```python
from build123d import *

# Parameters (mm, degrees)
SKETCH1_R               = 6.35
BOSS_EXTRUDE1_DEPTH     = 5.4
HORN_DEPTH              = 2.5
SKETCH4_R               = 1.4
CUT_EXTRUDE1_DEPTH      = 6.4
SKETCH5_R               = 0.5
CUT_EXTRUDE2_DEPTH      = 6.4
LPATTERN1_COUNT         = 4
LPATTERN1_PITCH         = 3
MIRROR1_COPY_1_SKETCH_R = 0.5
MIRROR1_COPY_1_DEPTH    = 6.4
MIRROR1_COPY_2_SKETCH_R = 0.5
MIRROR1_COPY_2_DEPTH    = 6.4
MIRROR1_COPY_3_SKETCH_R = 0.5
MIRROR1_COPY_3_DEPTH    = 6.4
CUT_EXTRUDE4_DEPTH      = 3
CIRPATTERN2_COUNT       = 26
SKETCH9_R               = 2.6
CUT_EXTRUDE5_DEPTH      = 3
SKETCH10_R              = 6.35
SKETCH10_R_2            = 4.25
CUT_EXTRUDE6_DEPTH      = 2.9
BOSS_EXTRUDE5_DEPTH     = 0.5
CIRPATTERN3_COUNT       = 4
SKETCH12_R              = 4.375
CUT_EXTRUDE7_DEPTH      = 1
SKETCH13_R              = 3.375
SKETCH13_R_2            = 2.875
BOSS_EXTRUDE6_DEPTH     = 1
SKETCH14_R              = 3.375
SKETCH14_R_2            = 2.875
BOSS_EXTRUDE7_DEPTH     = 0.35


with BuildPart() as part:
    # Sketch1 → Boss-Extrude1 (new body)
    with BuildSketch(Plane(origin=(0, 0, 0), x_dir=(1, 0, 0), z_dir=(0, 1, 0))):
        Circle(SKETCH1_R)
    extrude(amount=BOSS_EXTRUDE1_DEPTH)

    # Sketch2 → horn (add)
    with BuildSketch(Plane(origin=(0, 5.4, 0), x_dir=(1, 0, 0), z_dir=(0, 1, 0))):
        with BuildLine():
            Line((-2.609740545, 16.990167671), (-4.891612682, 4.049027706))
            ThreePointArc((-4.891612682, 4.049027706), (0, 6.35), (4.891612682, 4.049027706))
            Line((4.891612682, 4.049027706), (2.609740545, 16.990167671))
            ThreePointArc((2.609740545, 16.990167671), (0, 19.18), (-2.609740545, 16.990167671))
        make_face()
    horn = extrude(amount=-HORN_DEPTH)

    # Sketch4 → Cut-Extrude1 (cut, through all)
    with BuildSketch(Plane(origin=(0, 5.4, 0), x_dir=(-1, 0, 0), z_dir=(0, -1, 0))):
        Circle(SKETCH4_R)
    extrude(amount=CUT_EXTRUDE1_DEPTH, mode=Mode.SUBTRACT)

    # Sketch5 → Cut-Extrude2 (cut, through all)
    with BuildSketch(Plane(origin=(0, 0, 0), x_dir=(-1, 0, 0), z_dir=(0, -1, 0))):
        with Locations((0, 16.53)):
            Circle(SKETCH5_R)
    cut_extrude2 = extrude(amount=-CUT_EXTRUDE2_DEPTH, mode=Mode.SUBTRACT)

    # LPattern1: Cut-Extrude2 ×4
    with Locations(*[(0, 0, i * LPATTERN1_PITCH) for i in range(1, LPATTERN1_COUNT)]):
        add(cut_extrude2, mode=Mode.SUBTRACT)

    # Mirror1: horn, Cut-Extrude2 across plane
    add(horn.mirror(Plane.XY))
    add(cut_extrude2.mirror(Plane.XY), mode=Mode.SUBTRACT)

    # Mirror1 copy 1 sketch → Mirror1 copy 1 (cut, through all)
    with BuildSketch(Plane(origin=(0, 0, -3), x_dir=(-1, 0, 0), z_dir=(0, -1, 0))):
        with Locations((0, -16.53)):
            Circle(MIRROR1_COPY_1_SKETCH_R)
    extrude(amount=-MIRROR1_COPY_1_DEPTH, mode=Mode.SUBTRACT)

    # Mirror1 copy 2 sketch → Mirror1 copy 2 (cut, through all)
    with BuildSketch(Plane(origin=(0, 0, -6), x_dir=(-1, 0, 0), z_dir=(0, -1, 0))):
        with Locations((0, -16.53)):
            Circle(MIRROR1_COPY_2_SKETCH_R)
    extrude(amount=-MIRROR1_COPY_2_DEPTH, mode=Mode.SUBTRACT)

    # Mirror1 copy 3 sketch → Mirror1 copy 3 (cut, through all)
    with BuildSketch(Plane(origin=(0, 0, -9), x_dir=(-1, 0, 0), z_dir=(0, -1, 0))):
        with Locations((0, -16.53)):
            Circle(MIRROR1_COPY_3_SKETCH_R)
    extrude(amount=-MIRROR1_COPY_3_DEPTH, mode=Mode.SUBTRACT)

    # Sketch8 → Cut-Extrude4 (cut)
    with BuildSketch(Plane(origin=(0, 0, 0), x_dir=(-1, 0, 0), z_dir=(0, -1, 0))):
        with BuildLine():
            Line((0, -2.9), (0.262912611, -2.586672952))
            ThreePointArc((0.262912611, -2.586672952), (0, -2.6), (-0.262912611, -2.586672952))
            Line((-0.262912611, -2.586672952), (0, -2.9))
        make_face()
    cut_extrude4 = extrude(amount=-CUT_EXTRUDE4_DEPTH, mode=Mode.SUBTRACT)

    # CirPattern2: Cut-Extrude4 ×26 about axis
    cirpattern2_axis = Axis((0, 0, 0), (0, 1, 0))
    for i in range(1, CIRPATTERN2_COUNT):
        add(cut_extrude4.rotate(cirpattern2_axis, i * 360 / CIRPATTERN2_COUNT), mode=Mode.SUBTRACT)

    # Sketch9 → Cut-Extrude5 (cut)
    with BuildSketch(Plane(origin=(0, 0, 0), x_dir=(-1, 0, 0), z_dir=(0, -1, 0))):
        Circle(SKETCH9_R)
    extrude(amount=-CUT_EXTRUDE5_DEPTH, mode=Mode.SUBTRACT)

    # Sketch10 → Cut-Extrude6 (cut)
    with BuildSketch(Plane(origin=(0, 0, 0), x_dir=(-1, 0, 0), z_dir=(0, -1, 0))):
        Circle(SKETCH10_R)
        Circle(SKETCH10_R_2, mode=Mode.SUBTRACT)
    extrude(amount=-CUT_EXTRUDE6_DEPTH, mode=Mode.SUBTRACT)

    # Sketch11 → Boss-Extrude5 (add, symmetric)
    with BuildSketch(Plane.XY):
        Polygon((4.21, 0.99), (5.812680296, 2.9), (4.21, 2.9), (4.16, 2.9), (4.16, 0.99), align=None)
    boss_extrude5 = extrude(amount=BOSS_EXTRUDE5_DEPTH, both=True)

    # CirPattern3: Boss-Extrude5 ×4 about axis
    cirpattern3_axis = Axis((0, 0, 0), (0, 1, 0))
    for i in range(1, CIRPATTERN3_COUNT):
        add(boss_extrude5.rotate(cirpattern3_axis, i * 360 / CIRPATTERN3_COUNT))

    # Sketch12 → Cut-Extrude7 (cut)
    with BuildSketch(Plane(origin=(0, 5.4, 0), x_dir=(1, 0, 0), z_dir=(0, 1, 0))):
        Circle(SKETCH12_R)
    extrude(amount=-CUT_EXTRUDE7_DEPTH, mode=Mode.SUBTRACT)

    # Sketch13 → Boss-Extrude6 (add)
    with BuildSketch(Plane(origin=(0, 4.4, 0), x_dir=(1, 0, 0), z_dir=(0, 1, 0))):
        Circle(SKETCH13_R)
        Circle(SKETCH13_R_2, mode=Mode.SUBTRACT)
    extrude(amount=BOSS_EXTRUDE6_DEPTH)

    # Sketch14 → Boss-Extrude7 (add)
    with BuildSketch(Plane(origin=(0, 5.4, 0), x_dir=(1, 0, 0), z_dir=(0, 1, 0))):
        Circle(SKETCH14_R)
        Circle(SKETCH14_R_2, mode=Mode.SUBTRACT)
    extrude(amount=BOSS_EXTRUDE7_DEPTH)


solid = part.part
```
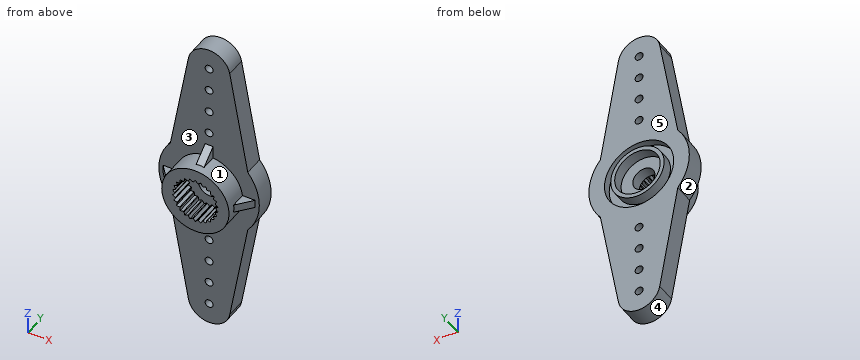
CAD build for the part. Positions are in the model's coordinates, mm. Face numbers are marked on the shaded views. A direction names the side the tool comes from. Round coordinates to 2 decimals unless told otherwise and drop trailing zeros. Loops run counter-clockwise (first coordinate to the right, second up) from the corner with the lowest first, then second, coordinate; pieces in that order, holes last. Notation, with made-up numbers: (33.5, 19.5) - (56.5, 19.5) arc R23 cw to (56.5, 32.5) - close; hole circle Ø9 at (36.5, 6). An arc over 180 degrees is marked (long way). Return JSON: item names as keys, results as strings. Group by question number.
Q1. Flat gauge pins, fed straight in: pin 1 Ø0.5 at (x, y) = (5.5, 2) entering from +Z; pin 2 Ø0.8 at (x, y) = (-5.5, 2) entering from -Z; pin 3 Ø3 at (x, z) = (-4, 11) entering from +Y; pin 4 Ø2 at (y, z) = (4.5, -13.5) entering from +X. Where does each tip first touch, or does it go through?
Q2. Band-saw the part on A-A on z = -7.53. Give the cut face in (x, y), plus the area to 3 significant figures.
Q3. Tool access for the marked faces 1 and 2: list every direction of +Z, -Z, +X, -X, +Y, -Y with a clear straight run to the whole face (end or side of a thin tool).
Q4. Band-saw the part on B-B on x = -5.25. Give the cut face in (y, z), plus the area to 3 significant figures.
Q5. Drill centre lines: line 1 along Z through (x, y) = (1, 5.35); line 2 along Y through (x, z) = (-1.5, 6); line 3 along Z through (x, y) = (-0.5, 0.85). Where is each one in solid material? Low to high. Write a range as [from, to].
Q6. Two-plate mould, pull along Y, no slides. Class the marked faces 3, 4 and 5: +Y half, -Y half, draft (parallel to the pull), parting line (faces both ways), or undercut.
Solutions:
{
 "1": {"pin 1": "passes through", "pin 2": "stops at z = -0.5", "pin 3": "stops at y = 5.4", "pin 4": "stops at x = 3.4"},
 "2": {"outline": "(-4.28, 2.9) - (-0.5, 2.9) - (-0.5, 5.4) - (-4.28, 5.4) - close; (0.5, 2.9) - (4.28, 2.9) - (4.28, 5.4) - (0.5, 5.4) - close", "area": "18.9 mm^2"},
 "3": {"face 1": "-Y", "face 2": "-X, +Y, -Y"},
 "4": {"outline": "(2.23, -0.5) - (2.9, -0.5) - (2.9, -3.57) - (5.4, -3.57) - (5.4, 3.57) - (2.9, 3.57) - (2.9, 0.5) - (2.23, 0.5) - close", "area": "18.5 mm^2"},
 "5": {"line 1": "z = [-18.98, -4.26], [-3.22, -2.7], [2.7, 3.22], [4.26, 18.98]", "line 2": "y = [2.9, 5.4]", "line 3": "z = [-4.22, -2.67], [2.67, 4.22]"},
 "6": {"face 3": "-Y half", "face 4": "draft", "face 5": "+Y half"}
}
